Build history of the part. All positions in model axes, mm. A direction names the side the tool comes from. Round coordinates to 2 decimals unless told otherwise and drop trailing zeros.
Autodesk Inventor part; units mm, degrees
ref_plane "YZ Plane" through (0, 0, 0) normal (1, 0, 0) x (0, 1, 0)
ref_plane "XZ Plane" through (0, 0, 0) normal (0, 1, 0) x (-1, 0, 0)
ref_plane "XY Plane" through (0, 0, 0) normal (0, 0, 1) x (1, 0, 0)
sketch "Sketch1" plane through (0, 0, 0) normal (0, 0, 1) x (1, 0, 0)
  line L0 (-5.1073, 0) -> (106.1447, 0)
  line L1 (106.1447, 0) -> (106.1447, 15.875)
  line L2 (106.1447, 15.875) -> (-5.1073, 15.875)
  line L3 (-5.1073, 15.875) -> (-5.1073, 0)
  point P0 (0, 0)
  dimension "d0" = 111.252
  dimension "d1" = 15.875
extrude "Extrusion1" add sketch "Sketch1" along normal blind 12.7
sketch "Sketch2" plane through (0, 0, 12.7) normal (0, 0, 1) x (1, 0, 0)
  line L0 (106.1447, 15.875) -> (-5.1073, 15.875)
  line L1 (12.8596, 15.875) -> (14.6926, 11.0998)
  line L2 (-5.1073, 0) -> (106.1447, 0)
  line L3 (14.6926, 11.0998) -> (16.2166, 11.0998)
  line L4 (16.2166, 11.0998) -> (18.0497, 15.875)
  point P0 (0, 0)
  dimension "d4" = 17.9669
  dimension "d5" = 11.0998
  dimension "d6" = 11.0998
  dimension "d10" = 42
  dimension "d11" = 1.524
extrude "Extrusion2" cut sketch "Sketch2" against normal blind 12.7
pattern_linear "Rectangular Pattern1" count 12 spacing 6.4516 along (1, 0, 0) of "Extrusion2"
chamfer "Chamfer1" distance 1.524 angle 45 4 edges at (106.1447, 7.9375, 12.7) (106.1447, 15.875, 6.35) (106.1447, 7.9375, 0) (106.1447, 0, 6.35)
sketch "Sketch3" plane through (-5.1073, 0, 0) normal (-1, 0, 0) x (0, 0, 1)
  circle A0 centre (6.35, 7.9248) radius 3.175
  line L0 (0, 15.875) -> (12.7, 15.875)
  line L1 (0, 15.875) -> (0, 0)
  dimension "d20" = 6.35
  dimension "d21" = 7.9502
  dimension "d22" = 6.35
extrude "Extrusion3" cut sketch "Sketch3" against normal blind 15.875
properties part number "Gear Rack" material "Stainless Steel"
(1) Which spindle directions (+Z, -Z, +X, -X, +Y, -Y) get a long thin tool onto all of the face, cutting with end or side? Do faces 5 (the face through (2.719, 5.993, 3.83)), 6 (the face through (55.83, 13.45, 6.44)). Say none if no direction does.
Responses:
face 5: -X
face 6: +Z, -Z, +Y
(2) Pull direction X, two halves, no side cores. Call faces 1 (the face through (10.768, 8, 6)), 2 (the face through (13.763, 13.521, 6.439)), 3 (the face through (106.145, 8, 6)), 4 (the face through (4, 15.875, 6)): +X half, -X half, draft (parallel to the pull), parting line (faces both ways), or undercut.
Responses:
face 1: -X half
face 2: undercut
face 3: +X half
face 4: draft
(3) Pin check, flat tips, straight feed: P1, Ø0.5, axis at x = 35, z = 5.5, coming from the +Y side; P2, Ø1.9, axis at y = 8.5, z = 5.5, coming from the -X side. Stop position of each tip, or through.
Responses:
P1: stops at y = 11.1
P2: stops at x = 10.77
(4) Probe line 1 (Y direction, x = 5, z = 6.35) (3 decimals); line 2 (Z direction, x = 2.5, y = 6); line 3 (X direction, y = 5.5, z = 7). List the from-to ranges inside material, lowest first.
Responses:
line 1: y = 0 to 4.75, 11.1 to 15.875
line 2: z = 0 to 3.82, 8.88 to 12.7
line 3: x = 10.77 to 106.14
